Could you check a few things on this model? Use its own coordinates, in mm. Face numbers are marked on the shaded views. Round coordinates to 2 decimals unless told otherwise and drop trailing zeros. Loops run counter-clockwise (first coordinate to the right, second up) from the corner with the lowest first, then second, coordinate; pieces in that order, holes last.
from build123d import *

# Parameters (mm, degrees)
SKETCH_1_R      = 10.25
SKETCH_1_R_2    = 1.5
EXTRUDE_1_DEPTH = 3.2
FILLET_1_R      = 1


with BuildPart() as part:
    # 草图1 → 凸台-拉伸1 (new body)
    with BuildSketch(Plane.XY):
        with BuildLine():
            Line((4.334015044, 74.86289651), (16.967477077, 63.487676201))
            ThreePointArc((16.967477077, 63.487676201), (17.955973862, 61.415249594), (17.189519734, 59.250849906))
            Line((17.189519734, 59.250849906), (7.944957082, 48.983722931))
            ThreePointArc((7.944957082, 48.983722931), (6.077132686, 47.683381281), (3.826448864, 47.345625871))
            ThreePointArc((3.826448864, 47.345625871), (-6.917114554, 46.993654106), (-17.306435746, 44.235023248))
            ThreePointArc((-17.306435746, 44.235023248), (-20.032995202, 43.973894607), (-22.488022071, 45.188455313))
            ThreePointArc((-22.488022071, 45.188455313), (-27.335046982, 51.900262342), (-29.048597084, 60))
            Line((-29.048597084, 60), (-29.048597084, 77))
            ThreePointArc((-29.048597084, 77), (-28.169917427, 79.121320344), (-26.048597084, 80))
            Line((-26.048597084, 80), (-9.048597084, 80))
            ThreePointArc((-9.048597084, 80), (-1.881238093, 78.67160853), (4.334015044, 74.86289651))
        make_face()
        with Locations((-9.048597084, 60)):
            Circle(SKETCH_1_R, mode=Mode.SUBTRACT)
        with Locations((-25.048597084, 76)):
            Circle(SKETCH_1_R_2, mode=Mode.SUBTRACT)
        with Locations((-3.314709891, 74.937286824)):
            Circle(SKETCH_1_R_2, mode=Mode.SUBTRACT)
        with Locations((-25.048597084, 60)):
            Circle(SKETCH_1_R_2, mode=Mode.SUBTRACT)
        with Locations((-19.128165824, 48.891341485)):
            Circle(SKETCH_1_R_2, mode=Mode.SUBTRACT)
        with Locations((4.229232955, 52.329375962)):
            Circle(SKETCH_1_R_2, mode=Mode.SUBTRACT)
        with Locations((13.547809826, 61.184227506)):
            Circle(SKETCH_1_R_2, mode=Mode.SUBTRACT)
    extrude(amount=EXTRUDE_1_DEPTH)

    # 圆角1
    fillet_1_edges = [part.edges().sort_by_distance(p)[0] for p in [
        (-29.048597084, 68.5, 0),
        (-28.169917427, 79.121320344, 0),
        (-17.548597084, 80, 0),
        (-1.881238093, 78.67160853, 0),
        (10.65074606, 69.175286355, 0),
        (17.955973862, 61.415249594, 0),
        (12.567238408, 54.117286418, 0),
        (6.077132686, 47.683381281, 0),
        (-6.917114554, 46.993654106, 0),
        (-20.032995202, 43.973894607, 0),
        (-27.335046982, 51.900262342, 0),
    ]]
    fillet(fillet_1_edges, radius=FILLET_1_R)


solid = part.part
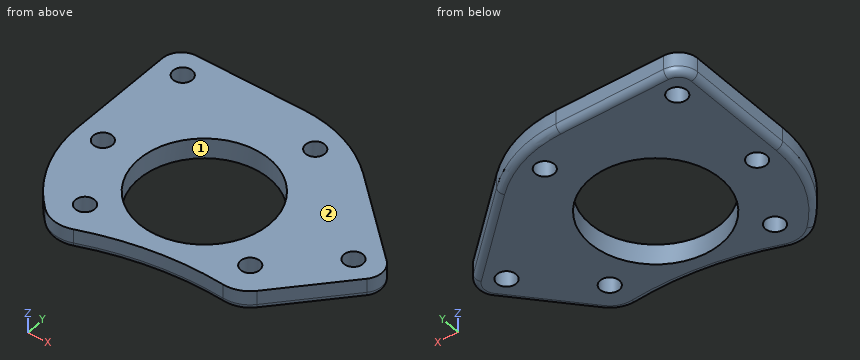
Item 1: If I drill on line 1 along X through (y, z) = (75, 2.8); line 2 along X through (y, z) = (76, 1.7); line 3 along Y through (x, z) = (-3.5, 0.8), over which ranges is the centre line in solid material (lowest first)?
Results list:
line 1: x = -29.05 to -26.17, -23.93 to -4.81, -1.82 to 4.18
line 2: x = -29.05 to -26.55, -23.55 to -4.37, -2.26 to 2.95
line 3: y = 47.39 to 51.38, 68.62 to 73.45, 76.43 to 79.19
Item 2: We'd pull the mould along X, two halves only. Please class the marked faces 1 and 2: released by +X, released by -X, zero draft, split by the parting line, or undercut.
Results list:
face 1: undercut
face 2: zero draft
Item 3: If we section it at B-B, the plane x = -3.5: Count the separate pieces of the cut face and the enclosed holes in it, then the cut area to 3 significant figures.
Results list:
separate pieces: 3
enclosed holes: 0
area: 36.8 mm2
Item 4: Will this pin go through, and if not, where does the flat tip stop? pin 1 (2.5 mm diameter, centred on x = -25.05, y = 76, fed in from -Z).
Results list:
pin 1: passes through
Item 5: If we section it at A-A, the plane z = 1.8: Please give me the cut outline in (x, y), then the cut area to 3 significant figures.
Results list:
outline: (-29.05, 60) arc R20 ccw to (-22.49, 45.19) arc R5 ccw to (-17.31, 44.24) arc R47.5 cw to (3.83, 47.35) arc R5 ccw to (7.94, 48.98) - (17.19, 59.25) arc R3 ccw to (16.97, 63.49) - (4.33, 74.86) arc R20 ccw to (-9.05, 80) - (-26.05, 80) arc R3 ccw to (-29.05, 77) - close; hole circle Ø3 at (-25.05, 60); hole circle Ø3 at (-25.05, 76); hole circle Ø3 at (-19.13, 48.89); hole circle Ø20.5 at (-9.05, 60); hole circle Ø3 at (-3.31, 74.94); hole circle Ø3 at (4.23, 52.33); hole circle Ø3 at (13.55, 61.18)
area: 927 mm2
